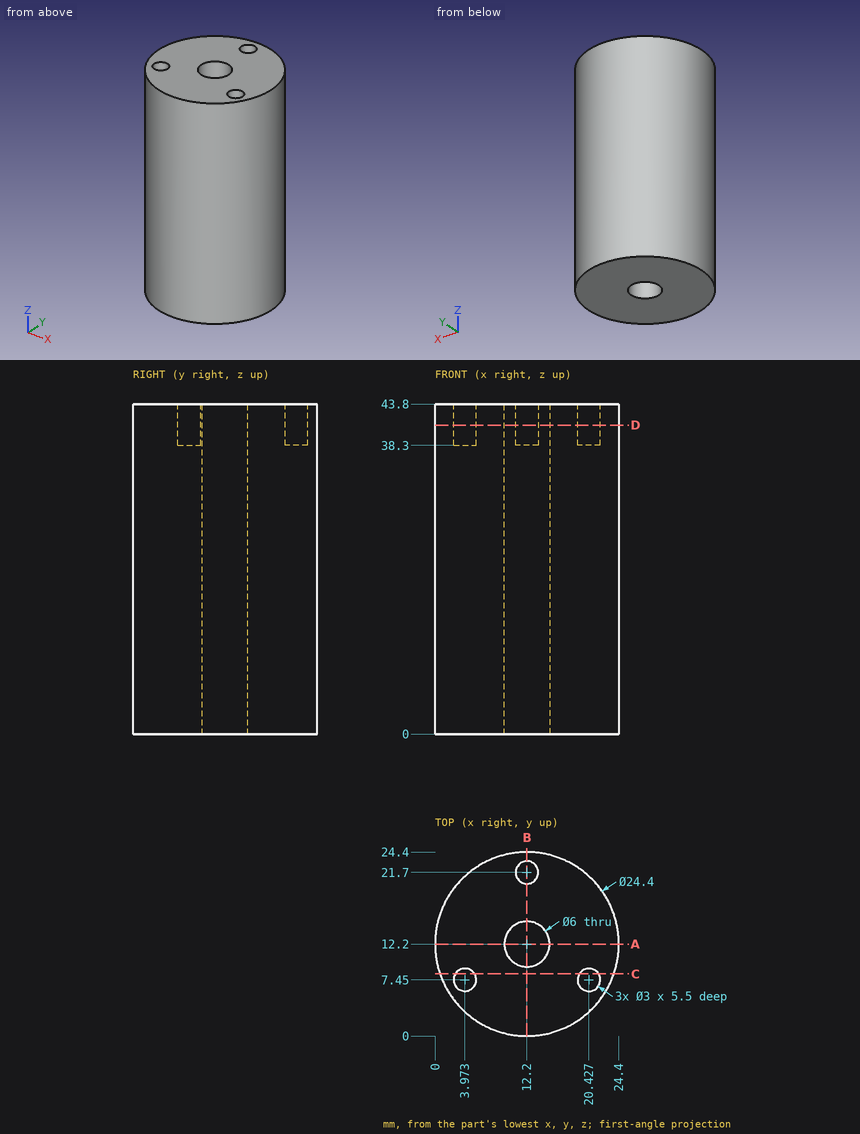
Geometry: see drawing. Coordinates: mm, zero at the bounding-box minimum. Coordinates: 2 decimals unless noted, no trailing zeros. Loops run counter-clockwise (first coordinate to the right, second up) from the corner with the lowest first, then second, coordinate; pieces in that order, holes last.
Q1. Cut plane B-B (x = 12.2). Output: boundary loops of the cut face in (y, z).
Q2. Material intervals for line 1 (Y direction, x = 12, z = 4); line 2 (Y direction, x = 12.2, z = 42.25); line 3 (X direction, y = 7.45, z = 42.7), sorted ascending.
Q3. Cut plane D-D (z = 41). Output: boundary loops of the cut face in (x, y).
Q4. Contact query for flat-ended pins moving along their axis: pin 1 (12 mm diameter, centred on y = 20, z = 22, fed in from -X); pin 2 (2 mm diameter, centred on y = 17, z = 30.5, fed in from +X); pin 3 (1 mm diameter, centred on x = 21, z = 17.5, fed in from +Y). Output: stop coordinate, or through.
Q5. Cut plane A-A (y = 12.2). Output: boundary loops of the cut face in (x, z), then the cut area to 3 significant figures.
Q6. Cut plane C-C (y = 8.25). Output: boundary loops of the cut face in (x, z).
Working result:
1. outline: (0, 0) - (9.2, 0) - (9.2, 43.8) - (0, 43.8) - close; (15.2, 0) - (24.4, 0) - (24.4, 43.8) - (23.2, 43.8) - (23.2, 38.3) - (20.2, 38.3) - (20.2, 43.8) - (15.2, 43.8) - close
2. line 1: y = 0 to 9.21, 15.19 to 24.4
2. line 2: y = 0 to 9.2, 15.2 to 20.2, 23.2 to 24.4
2. line 3: x = 0.96 to 2.47, 5.47 to 18.93, 21.93 to 23.44
3. outline: circle Ø24.4 at (12.2, 12.2); hole circle Ø3 at (3.97, 7.45); hole circle Ø6 at (12.2, 12.2); hole circle Ø3 at (12.2, 21.7); hole circle Ø3 at (20.43, 7.45)
4. pin 1: stops at x = 0.13
4. pin 2: stops at x = 23.79
4. pin 3: stops at y = 21.14
5. outline: (0, 0) - (9.2, 0) - (9.2, 43.8) - (0, 43.8) - close; (15.2, 0) - (24.4, 0) - (24.4, 43.8) - (15.2, 43.8) - close
5. area: 806 mm2
6. outline: (0.66, 0) - (23.74, 0) - (23.74, 43.8) - (21.7, 43.8) - (21.7, 38.3) - (19.16, 38.3) - (19.16, 43.8) - (5.24, 43.8) - (5.24, 38.3) - (2.7, 38.3) - (2.7, 43.8) - (0.66, 43.8) - close
